from build123d import *

# Parameters (mm, degrees)
SKETCH1_W           = 47
SKETCH1_H           = 17
BOSS_EXTRUDE1_DEPTH = 1.5
SKETCH3_W           = 21
SKETCH3_H           = 17
SKETCH3_W_2         = 4
SKETCH3_H_2         = 2
BOSS_EXTRUDE3_DEPTH = 2
SKETCH2_W           = 50.2
SKETCH2_H           = 20.2
SKETCH2_W_2         = 47
SKETCH2_H_2         = 17
BOSS_EXTRUDE2_DEPTH = 8.5
SKETCH4_W           = 3
SKETCH4_H           = 8
CUT_EXTRUDE1_DEPTH  = 2.6


with BuildPart() as part:
    # Sketch1 → Boss-Extrude1 (new body)
    with BuildSketch(Plane.XY):
        Rectangle(SKETCH1_W, SKETCH1_H)
    extrude(amount=BOSS_EXTRUDE1_DEPTH)

    # Sketch3 → Boss-Extrude3 (add)
    with BuildSketch(Plane.XY.offset(1.5)):
        with Locations((-13, 0)):
            Rectangle(SKETCH3_W, SKETCH3_H)
        with Locations((21.5, 7.5)):
            Rectangle(SKETCH3_W_2, SKETCH3_H_2)
        with Locations((21.5, -7.5)):
            Rectangle(SKETCH3_W_2, SKETCH3_H_2)
    extrude(amount=BOSS_EXTRUDE3_DEPTH)

    # Sketch2 → Boss-Extrude2 (add)
    with BuildSketch(Plane.XY):
        Rectangle(SKETCH2_W, SKETCH2_H)
        Rectangle(SKETCH2_W_2, SKETCH2_H_2, mode=Mode.SUBTRACT)
    extrude(amount=BOSS_EXTRUDE2_DEPTH)

    # Sketch4 → Cut-Extrude1 (cut, through all)
    with BuildSketch(Plane(origin=(-23.5, 0, 0), x_dir=(0, 0, -1), z_dir=(1, 0, 0))):
        with Locations((-5, 0)):
            Rectangle(SKETCH4_W, SKETCH4_H)
    extrude(amount=-CUT_EXTRUDE1_DEPTH, mode=Mode.SUBTRACT)


solid = part.part
Design review of the part built by this model. Coordinates are the model's own, in mm. A direction names the side the tool comes from. Round coordinates to 2 decimals unless told otherwise and drop trailing zeros. Write each loop counter-clockwise with the first axis right and the second up, starting at its lowest first coordinate (ties: lowest second). Pieces come first, ordered by that corner, then holes. Notation, with made-up numbers: (-35.75, 79) - (-9.75, 79) arc R19 ccw to (-9.75, 91) - close; hole circle Ø10 at (78, 9). An arc over 180 degrees is marked (long way). Use a Markdown table: item, result. Add a question column.
1. We need section D-D (z = 5.25). State the section outline as (x, y) points, then the cut area to 3 significant figures.
2. We need section B-B (y = 2). State the section outline as (x, z) points, then the cut area to 3 significant figures.
3. We need section C-C (x = 18). State the section outline as (y, z) points, then the cut area to 3 significant figures.
4. Wall thickness on probe 1 along X at (y, z) = (-7.5, 5); probe 2 along Y at (x, z) = (10, 7); probe 3 along X at (y, z) = (-8.25, 2.25): over which ranges is each line inside the solid? List them lowest first.
5. We need section A-A (z = 2.25). State the section outline as (x, y) points, then the cut area to 3 significant figures.
6. For faces 5 (the face through (23.5, 0, 5)), 6 (the face through (-2, -9, 8.5)), list the 3-axis set-ups (+Z, -Z, +X, -X, +Y, -Y) from which the entire face can be reached by the end or side of a thin tool; tool diameter is ignored.
7. Clearance check with flat-ended pins moving along their axes: pin 1 (1.3 mm diameter, centred on x = -24.5, y = 1.5, fed in from -Z); pin 2 (2 mm diameter, centred on x = 20.5, y = 7, fed in from +Z); pin 3 (10 mm diameter, centred on x = 7.5, y = -1.5, fed in from +Z). State where each tip first meets the part, or that it passes through.
8. Mouldability with a two-part tool opening along Z and no side actions: class faces 1 (the face through (0, 0, 0)), 2 (the face through (-24, -4, 5)), 3 (the face through (19.5, 7, 2)), 4 (the face through (-24, 0, 6.5)) as +Z half, -Z half, draft (parallel to the pull), parting line (faces both ways), or undercut.
Output:
| question | item | result |
|---|---|---|
| 1 | outline | (-25.1, -10.1) - (25.1, -10.1) - (25.1, 10.1) - (-25.1, 10.1) - (-25.1, 4) - (-23.5, 4) - (-23.5, 8.5) - (23.5, 8.5) - (23.5, -8.5) - (-23.5, -8.5) - (-23.5, -4) - (-25.1, -4) - close |
| 1 | area | 202 mm2 |
| 2 | outline | (-25.1, 0) - (25.1, 0) - (25.1, 8.5) - (23.5, 8.5) - (23.5, 1.5) - (-2.5, 1.5) - (-2.5, 3.5) - (-25.1, 3.5) - close; (-25.1, 6.5) - (-23.5, 6.5) - (-23.5, 8.5) - (-25.1, 8.5) - close |
| 2 | area | 135 mm2 |
| 3 | outline | (-10.1, 0) - (10.1, 0) - (10.1, 8.5) - (8.5, 8.5) - (8.5, 1.5) - (-8.5, 1.5) - (-8.5, 8.5) - (-10.1, 8.5) - close |
| 3 | area | 52.7 mm2 |
| 4 | probe 1 | x = -25.1 to -23.5, 23.5 to 25.1 |
| 4 | probe 2 | y = -10.1 to -8.5, 8.5 to 10.1 |
| 4 | probe 3 | x = -25.1 to -2.5, 19.5 to 25.1 |
| 5 | outline | (-25.1, -10.1) - (25.1, -10.1) - (25.1, 10.1) - (-25.1, 10.1) - close; hole (-2.5, -8.5) - (19.5, -8.5) - (19.5, -6.5) - (23.5, -6.5) - (23.5, 6.5) - (19.5, 6.5) - (19.5, 8.5) - (-2.5, 8.5) - close |
| 5 | area | 588 mm2 |
| 6 | face 5 | +Z |
| 6 | face 6 | +Z, +X, -X, +Y, -Y |
| 7 | pin 1 | stops at z = 0 |
| 7 | pin 2 | stops at z = 3.5 |
| 7 | pin 3 | stops at z = 1.5 |
| 8 | face 1 | -Z half |
| 8 | face 2 | undercut |
| 8 | face 3 | draft |
| 8 | face 4 | undercut |
